Design review of the part shown in the three views and the two pictorial views. Dimensions are in mm from the part's minimum x, y and z. A direction names the side the tool comes from. Give positions to 0.01 mm unless a question says otherwise; leave off trailing zeros. Write each loop counter-clockwise with the first axis right and the second up, starting at its lowest first coordinate (ties: lowest second). Pieces come first, ordered by that corner, then holes. Notation, with made-up numbers: (80.25, -9) -> (111.25, -9) arc R31 ccw to (111.25, 30) -> close; hole circle Ø2 at (88.5, 54). An arc over 180 degrees is marked (long way). Use CSV: the item, a comma, the result in double quotes.
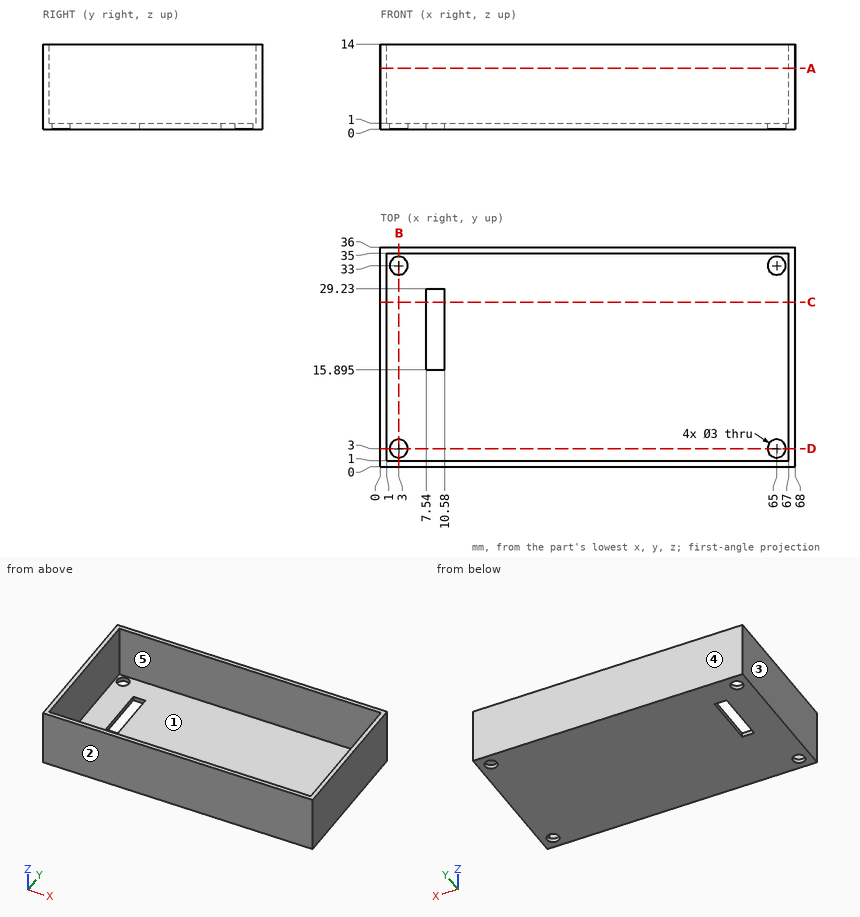
Q1. Consider section D-D (y = 3). Write out the cut boundary in (x, z).
Derived:
outline,"(0, 0) -> (1.5, 0) -> (1.5, 1) -> (1, 1) -> (1, 14) -> (0, 14) -> close; (4.5, 0) -> (63.5, 0) -> (63.5, 1) -> (4.5, 1) -> close; (66.5, 0) -> (68, 0) -> (68, 14) -> (67, 14) -> (67, 1) -> (66.5, 1) -> close"
Q2. Consider section A-A (z = 10). Write out the cut boundary in (x, y).
Derived:
outline,"(0, 0) -> (68, 0) -> (68, 36) -> (0, 36) -> close; hole (1, 1) -> (67, 1) -> (67, 35) -> (1, 35) -> close"
Q3. Insertion check: pin 1 (3 mm diameter, centred on x = 20, y = 23.5, fed in from +Z). The pin has a flat end and moves straight along its axis. Give the tip position at first contact, or say it passes through.
Derived:
pin 1,"stops at z = 1"
Q4. To check wall thickness, follow probe 1 along Y at (x, z) = (3, 0.75); probe 2 along Y at (x, z) = (32, 2.5); probe 3 along X at (y, z) = (19, 10.25). State the ranges of each line that lie inside material, in increasing order.
Derived:
probe 1,"y = 0 to 1.5, 4.5 to 31.5, 34.5 to 36"
probe 2,"y = 0 to 1, 35 to 36"
probe 3,"x = 0 to 1, 67 to 68"
Q5. The part is to be moulded in two halves that separate along X. For the marked faces 3, 4 and 5, say which applies: pulls with the +X half, pulls with the -X half, needs draft (parallel to the pull), parting line crosses it, or undercut.
Derived:
face 3,"pulls with the -X half"
face 4,"needs draft"
face 5,"undercut"
Q6. Consider section B-B (x = 3). Write out the cut boundary in (y, z), then the cut area to 3 significant figures.
Derived:
outline,"(0, 0) -> (1.5, 0) -> (1.5, 1) -> (1, 1) -> (1, 14) -> (0, 14) -> close; (4.5, 0) -> (31.5, 0) -> (31.5, 1) -> (4.5, 1) -> close; (34.5, 0) -> (36, 0) -> (36, 14) -> (35, 14) -> (35, 1) -> (34.5, 1) -> close"
area,"56.0 mm2"
Q7. Machinability: for the marked faces 1 and 2, which of the approach directions +Z, -Z, +X, -X, +Y, -Y give a long, thin tool a straight path to every point of the face, cutting with its end or side? Answer none if there is none.
Derived:
face 1,"+Z"
face 2,"+Z, -Z, +X, -X, -Y"
Q8. Consider section C-C (y = 27). Write out the cut boundary in (x, z), then the cut area to 3 significant figures.
Derived:
outline,"(0, 0) -> (7.54, 0) -> (7.54, 1) -> (1, 1) -> (1, 14) -> (0, 14) -> close; (10.58, 0) -> (68, 0) -> (68, 14) -> (67, 14) -> (67, 1) -> (10.58, 1) -> close"
area,"91.0 mm2"
